Part print with two shaded views. Sizes in mm from the minimum x, y, z corner. Give positions to 0.01 mm unless a question says otherwise; leave off trailing zeros. Write each loop counter-clockwise with the first axis right and the second up, starting at its lowest first coordinate (ties: lowest second). Pieces come first, ordered by that corner, then holes. Notation, with made-up numbers: (52, 2.5) - (88, 2.5) arc R16 cw to (88, 29.5) - close; hole circle Ø2 at (31, -28.75). An arc over 180 degrees is marked (long way). One line per item, written item: value. Start each with the question number.
(1) Cut at B-B, the plane x = 36.5. List the corners of the cut face in (y, z), and give its area (3 significant figures).
(2) Cut at D-D, the plane y = 1. List the corners of the cut face in (x, z).
(3) Cut at A-A, the plane y = 7.25. List the corners of the cut face in (x, z), and give its area (3 significant figures).
(4) Drop flat-ended pins along their axis: P1, Ø0.6, axis at y = 1, z = 9, coming from the -X side; P2, Ø0.7, axis at y = 6, z = 24, coming from the -X side; P3, Ø0.6, axis at y = 0.5, z = 8, coming from the +X side. Give the stop position or say it passes through.
(5) Probe L1, parallel to X at y = 2.5, z = 36.5; L2, parallel to Y at x = 49, z = 42.5; L3, parallel to Y at x = 27.5, z = 3. List the from-to ranges inside material, lowest first.
(6) Cut at C-C, the plane z = 36.5. List the corners of the cut face in (x, y).
(7) Mould opens along X. For the marked faces 1 and 2 say: pulls with the +X half, pulls with the -X half, needs draft (parallel to the pull), parting line crosses it, or undercut.
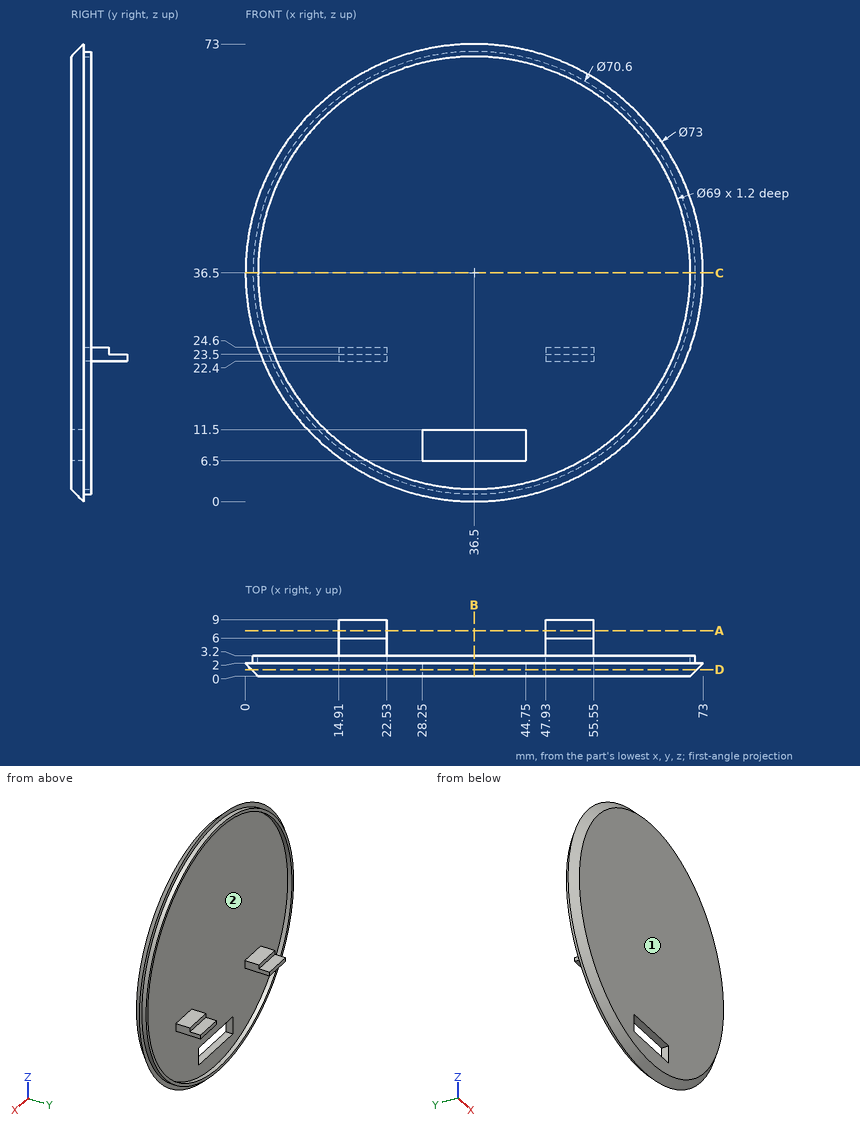
Answers follow:
1. outline: (0, 2) - (2, 0) - (2, 1.2) - (3.2, 1.2) - (3.2, 2) - (2, 2) - (2, 6.5) - (0, 6.5) - close; (0, 11.5) - (2, 11.5) - (2, 71) - (3.2, 71) - (3.2, 71.8) - (2, 71.8) - (2, 73) - (0, 71) - close
1. area: 134 mm²
2. outline: circle Ø71 at (36.5, 36.5); hole (28.25, 6.5) - (44.75, 6.5) - (44.75, 11.5) - (28.25, 11.5) - close
3. outline: (14.91, 22.4) - (22.53, 22.4) - (22.53, 23.5) - (14.91, 23.5) - close; (47.93, 22.4) - (55.55, 22.4) - (55.55, 23.5) - (47.93, 23.5) - close
3. area: 16.8 mm²
4. P1: stops at x = 13.46
4. P2: stops at x = 14.91
4. P3: stops at x = 57.47
5. L1: x = 1.2 to 2, 71 to 71.8
5. L2: y = 0 to 2
5. L3: y = 0.19 to 3.2
6. outline: (0, 2) - (2, 0) - (71, 0) - (73, 2) - (71.8, 2) - (71.8, 3.2) - (71, 3.2) - (71, 2) - (2, 2) - (2, 3.2) - (1.2, 3.2) - (1.2, 2) - close
7. face 1: needs draft
7. face 2: undercut
